from build123d import *

# Parameters (mm, degrees)
CYLINDER047_R     = 2
CYLINDER047_DEPTH = 10
CYLINDER048_R     = 2
CYLINDER048_DEPTH = 10
BOX_W             = 51
BOX_H             = 12.5
BOX_DEPTH         = 1.6


with BuildPart() as cylinder047:
    # Cylinder047 → Cylinder047 (new body)
    with BuildSketch(Plane(origin=(23, 2.5, 0), x_dir=(1, 0, 0), z_dir=(0, 0, 1))):
        Circle(CYLINDER047_R)
    extrude(amount=CYLINDER047_DEPTH)


with BuildPart() as fusion036:
    # Cylinder048 → Cylinder048 (new body)
    with BuildSketch(Plane(origin=(-23, 2.5, 0), x_dir=(1, 0, 0), z_dir=(0, 0, 1))):
        Circle(CYLINDER048_R)
    extrude(amount=CYLINDER048_DEPTH)

    # Fusion036: union Cylinder047
    add(cylinder047.part)


with BuildPart() as sensor:
    # Box → Box (new body)
    with BuildSketch(Plane(origin=(-25.5, 0, 0), x_dir=(1, 0, 0), z_dir=(0, 0, 1))):
        with Locations((25.5, 6.25)):
            Rectangle(BOX_W, BOX_H)
    extrude(amount=BOX_DEPTH)

    # Cut: cut Fusion036
    add(fusion036.part, mode=Mode.SUBTRACT)


with BuildPart() as sensor_1:
    # Cut placement: moved
    add(sensor.part.moved(Location((0, 139, -1.6))))


solid = sensor_1.part
The model under review builds one solid part; all positions refer to its coordinate system, in mm. Give positions to 0.01 mm unless a question says otherwise; leave off trailing zeros. Order: outer loops, then holes, each group sorted by start corner. A loop starts at its lowest first (then second) coordinate and runs counter-clockwise, first axis right, second up. Notation, with made-up numbers: M 60,-30 L 113,-30 A12 cw 113,-24 Z; hole C 66,-31 d10. An arc over 180 degrees is marked long. One line per question, with ' | ' between items. Start each with the question number.
1) Wall thickness on L1, parallel to X at y = 141.5, z = -0.5; L2, parallel to Y at x = -23, z = -1.15; L3, parallel to X at y = 140.5, z = -0.65: over which ranges is each line inside the solid? List them lowest first. Write a range as from..to.
2) Consider section C-C, the plane z = -0.25. Give the boundary of the cut face in (x, y), then the cut area to 3 significant figures.
3) Consider section B-B, the plane y = 141.5. Give the boundary of the cut face in (x, z), then the cut area to 3 significant figures.
4) Mouldability with a two-part tool opening along Y and no side actions: class faces 1 (the face through (0, 145, 0)), 2 (the face through (-22.077, 139.726, -0.811)), 3 (the face through (0, 151.5, -1)) as pulls with the +Y half, pulls with the -Y half, needs draft (parallel to the pull), parting line crosses it, or undercut.
5) Consider section A-A, the plane x = 23. Give the boundary of the cut face in (y, z).
6) Clearance check with flat-ended pins moving along their axes: P1, Ø2, axis at x = 6.5, y = 145.5, coming from the +Z side; P2, Ø3.5, axis at x = 23, y = 141.5, coming from the -Z side. State where each tip first meets the part, or that it passes through.
Found:
1) L1: x = -25.5..-25, -21..21, 25..25.5 | L2: y = 139..139.5, 143.5..151.5 | L3: x = -25.5..-24.73, -21.27..21.27, 24.73..25.5
2) outline: M -25.5,139 L 25.5,139 L 25.5,151.5 L -25.5,151.5 Z; hole C -23,141.5 d4; hole C 23,141.5 d4 | area: 612 mm²
3) outline: M -25.5,-1.6 L -25,-1.6 L -25,0 L -25.5,0 Z; M -21,-1.6 L 21,-1.6 L 21,0 L -21,0 Z; M 25,-1.6 L 25.5,-1.6 L 25.5,0 L 25,0 Z | area: 68.8 mm²
4) face 1: needs draft | face 2: undercut | face 3: pulls with the +Y half
5) outline: M 139,-1.6 L 139.5,-1.6 L 139.5,0 L 139,0 Z; M 143.5,-1.6 L 151.5,-1.6 L 151.5,0 L 143.5,0 Z
6) P1: stops at z = 0 | P2: passes through
